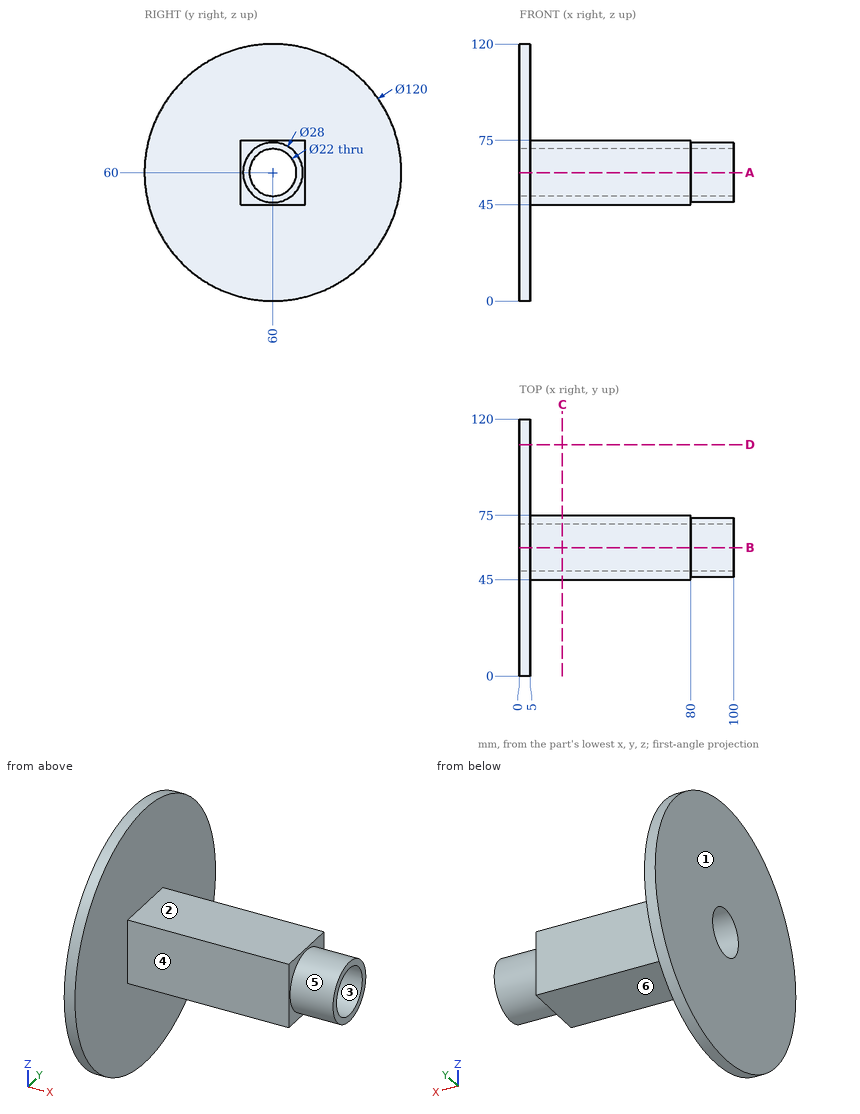
Study the drawing (mm; zero at the part's minimum x, y, z) and answer. A direction names the side the tool comes from. Coordinates: 2 decimals unless noted, no trailing zeros. Loops run counter-clockwise (first coordinate to the right, second up) from the corner with the lowest first, then second, coordinate; pieces in that order, holes last. Notation, with made-up numbers: M 66,-7.75 L 80,-7.75 A28 cw 80,26.25 Z; hole C -15,-18.75 d11. An arc over 180 degrees is marked long. Answer in a Markdown table with one row per item.
1) Determine the mould class of the marked faces 1, 2 and 3 for opening direction Z: released by +Z, released by -Z, zero draft, split by the parting line, or undercut.
Answers below:
| item | result |
|---|---|
| face 1 | zero draft |
| face 2 | released by +Z |
| face 3 | undercut |
2) Find section A-A (z = 60). Determine the outline of the cut face in (x, y), then the cut area to 3 significant figures.
Answers below:
| item | result |
|---|---|
| outline | M 0,0 L 5,0 L 5,45 L 80,45 L 80,46 L 100,46 L 100,49 L 0,49 Z; M 0,71 L 100,71 L 100,74 L 80,74 L 80,75 L 5,75 L 5,120 L 0,120 Z |
| area | 1,210 mm^2 |
3) Find section C-C (x = 20). Determine the outline of the cut face in (y, z).
Answers below:
| item | result |
|---|---|
| outline | M 45,45 L 75,45 L 75,75 L 45,75 Z; hole C 60,60 d22 |
4) Find section D-D (y = 108). Determine the outline of the cut face in (x, z), then the cut area to 3 significant figures.
Answers below:
| item | result |
|---|---|
| outline | M 0,24 L 5,24 L 5,96 L 0,96 Z |
| area | 360 mm^2 |
5) Given pin 1 (24 mm diameter, centred on y = 57.5, z = 60.5, fed in from +X); pin 2 (9 mm diameter, centred on x = 52.5, z = 57.5, fed in from -Y); pin 3 (10 mm diameter, centred on y = 78.5, z = 19, fed in from +X); pin 4 (20 mm diameter, centred on y = 60, z = 60, fed in from +X), each flat-ended and moving along its own axis, determine where each tip first touches the part or whether it passes through.
Answers below:
| item | result |
|---|---|
| pin 1 | x = 100 |
| pin 2 | y = 45 |
| pin 3 | x = 5 |
| pin 4 | through |
6) Which of the six approach directions +Z, -Z, +X, -X, +Y, -Y give full straight-line access (tool end or side, diameter ignored) to the marked faces 4, 5 and 6?
Answers below:
| item | result |
|---|---|
| face 4 | +Z, -Z, +X, -Y |
| face 5 | +X |
| face 6 | -Z, +X, +Y, -Y |
7) Find the intervals of material crossed by probe 1 along Z at (x, y) = (62, 60); probe 2 along X at (y, z) = (52, 17.5); probe 3 along Y at (x, z) = (29.5, 72), in increasing order.
Answers below:
| item | result |
|---|---|
| probe 1 | 45 to 49, 71 to 75 |
| probe 2 | 0 to 5 |
| probe 3 | 45 to 75 |
